Geometry check sheet. Reference: the model listing, model coordinates, mm. Face numbers are marked on the shaded views. A direction names the side the tool comes from. Coordinates: 2 decimals unless noted, no trailing zeros. Write each loop counter-clockwise with the first axis right and the second up, starting at its lowest first coordinate (ties: lowest second). Pieces come first, ordered by that corner, then holes. Notation, with made-up numbers: (35, 62) -> (82, 62) arc R31 cw to (82, 98) -> close; hole circle Ø3 at (-30, 65). An arc over 180 degrees is marked (long way). Answer in a Markdown table with one row per item. Add a question column.
1. Scan lines: L1, parallel to X at y = 678, z = -391.5; L2, parallel to Y at x = 440, z = -250; L3, parallel to Z at x = 704.5, y = 69.5. Record each from-to range of solid material in increasing order. Write a range as from..to.
2. Depth check by flat-ended pin: P1, Ø12, axis at x = 483, z = -215, coming from the +Y side; P2, Ø6, axis at x = 515, y = 307, coming from the -Z side; P3, Ø5, axis at x = 134, y = 323, coming from the -Z side. Enter the tip coordinate at first touch or a pass-through.
3. Mould release check, pull along X, two halves, no side actions. Record for the marked faces 3, 4 and 5: pulls with the +X half, pulls with the -X half, needs draft (parallel to the pull), parting line crosses it, or undercut.
4. Cross-section at A-A on x = 337. Record the cut outline in (y, z).
5. Cross-section at C-C on z = -74. Record the cut outline in (x, y).
6. Set-up check for the marked faces 1 and 2: record each of +Z, -Z, +X, -X, +Y, -Y from which the full face is reachable in a straight line by a thin tool's end or side.
7. Cross-section at B-B on y = 282. Record the cut outline in (x, z), and give its area (3 significant figures).
```python
from build123d import *

# Parameters (mm, degrees)
BOSS_EXTRUDE1_DEPTH = 762
BOSS_EXTRUDE2_DEPTH = 38.1


with BuildPart() as part:
    # Sketch1 → Boss-Extrude1 (new body)
    with BuildSketch(Plane(origin=(0, 0, 0), x_dir=(0, 0, -1), z_dir=(1, 0, 0))):
        Polygon((46.92577301, 408.932434185), (341.339964863, 487.820479132), (265.552255804, 770.66405993), (-127, 665.48), (-127, 0), (0, 0), (2.243845254, 332.732434185), align=None)
    extrude(amount=BOSS_EXTRUDE1_DEPTH)

    # Sketch3 → Loft1 section 0
    with BuildSketch(Plane(origin=(0, 770.66405993, 0), x_dir=(1, 0, 0), z_dir=(0, 1, 0))):
        with BuildLine():
            Line((762, 265.552255804), (762, 392.552255804))
            Line((762, 392.552255804), (736.6, 392.552255804))
            Line((736.6, 392.552255804), (635, 290.952255804))
            Line((635, 290.952255804), (635, 265.552255804))
            Line((635, 265.552255804), (762, 265.552255804))
        make_face()
    # Sketch4 → Loft1 section 1
    with BuildSketch(Plane(origin=(0, 525.920479132, 0), x_dir=(1, 0, 0), z_dir=(0, 1, 0))):
        with BuildLine():
            Line((762, 331.131100631), (762, 585.131100631))
            Line((762, 585.131100631), (736.6, 585.131100631))
            Line((736.6, 585.131100631), (533.4, 356.531100631))
            Line((533.4, 356.531100631), (533.4, 331.131100631))
            Line((533.4, 331.131100631), (762, 331.131100631))
        make_face()
    loft1 = loft()

    # Sketch4<5> → Boss-Extrude2 (add)
    with BuildSketch(Plane(origin=(0, 525.920479132, 0), x_dir=(1, 0, 0), z_dir=(0, 1, 0))):
        Polygon((762, 331.131100631), (762, 585.131100631), (736.6, 585.131100631), (533.4, 356.531100631), (533.4, 331.131100631), align=None)
    boss_extrude2 = extrude(amount=-BOSS_EXTRUDE2_DEPTH)

    # Mirror1: Loft1, Boss-Extrude2 across plane
    add(loft1.mirror(Plane(origin=(381, 0, 0), x_dir=(0, 0, 1), z_dir=(1, 0, 0))))
    add(boss_extrude2.mirror(Plane(origin=(381, 0, 0), x_dir=(0, 0, 1), z_dir=(1, 0, 0))))


solid = part.part
```
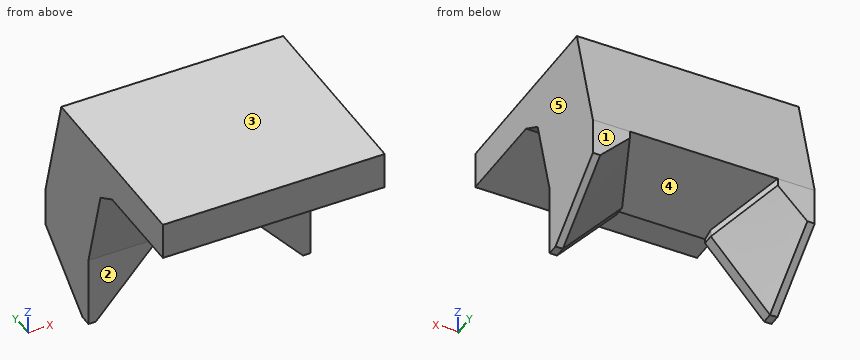
Results found:
| question | item | result |
|---|---|---|
| 1 | L1 | x = 0..94.61, 667.39..762 |
| 1 | L2 | y = 463.35..766.5 |
| 1 | L3 | z = -0.47..127 |
| 2 | P1 | stops at y = 758.73 |
| 2 | P2 | stops at z = -2.09 |
| 2 | P3 | stops at z = -2.2 |
| 3 | face 3 | needs draft |
| 3 | face 4 | undercut |
| 3 | face 5 | pulls with the +X half |
| 4 | outline | (0, 0) -> (332.73, -2.24) -> (408.93, -46.93) -> (487.82, -341.34) -> (770.66, -265.55) -> (665.48, 127) -> (0, 127) -> close |
| 5 | outline | (0, 416.19) -> (762, 416.19) -> (762, 719.34) -> (0, 719.34) -> close |
| 6 | face 1 | +Z, -Z, +X, -X, +Y |
| 6 | face 2 | -Z, +X, -X, -Y |
| 7 | outline | (0, -1.9) -> (762, -1.9) -> (762, 127) -> (0, 127) -> close |
| 7 | area | 98,200 mm^2 |
